from build123d import *

# Parameters (mm, degrees)
SKETCH1_R               = 16.6751
BOSS_EXTRUDE1_DEPTH     = 79.375
CUT_EXTRUDE1_DEPTH      = 83.804037009
CUT_EXTRUDE1_DEPTH_BACK = 83.804037009
SKETCH1_4_R             = 10.4648
SKETCH1_5_R             = 13.4366
SKETCH1_5_R_2           = 10.4648
CUT_EXTRUDE2_DEPTH      = 18.288
CUT_EXTRUDE3_START      = -18.288
SKETCH2_R               = 13.4366
SKETCH2_R_2             = 10.4648
CUT_EXTRUDE3_DEPTH      = 18.288
SKETCH3_R               = 13.5001
BOSS_EXTRUDE2_DEPTH     = 31.75
SKETCH3_7_R             = 7.8994
CUT_EXTRUDE5_DEPTH      = 33.3502
CUT_EXTRUDE6_START      = -17.526
SKETCH4_R               = 10.7696
SKETCH4_R_2             = 7.8994
CUT_EXTRUDE6_DEPTH      = 17.526
FILLET1_R               = 2.54


with BuildPart() as part:
    # Sketch1 → Boss-Extrude1 (new body)
    with BuildSketch(Plane(origin=(0, 0, 0), x_dir=(1, 0, 0), z_dir=(0, 1, 0))):
        with Locations(Location((0, 0, 0), (0, 0, 90))):
            Circle(SKETCH1_R)
    extrude(amount=BOSS_EXTRUDE1_DEPTH)

    # Sketch1<4> → Cut-Extrude1 (cut, two sides: drawn at the far end of the back side and taken through both)
    with BuildSketch(Plane(origin=(0, 0, 0), x_dir=(1, 0, 0), z_dir=(0, 1, 0)).offset(-CUT_EXTRUDE1_DEPTH_BACK)):
        with Locations(Location((0, 0, 0), (0, 0, 90))):
            Circle(SKETCH1_4_R)
    extrude(amount=CUT_EXTRUDE1_DEPTH + CUT_EXTRUDE1_DEPTH_BACK, mode=Mode.SUBTRACT)

    # Sketch1<5> → Cut-Extrude2 (cut)
    with BuildSketch(Plane(origin=(0, 0, 0), x_dir=(1, 0, 0), z_dir=(0, 1, 0))):
        with Locations(Location((0, 0, 0), (0, 0, 270))):
            Circle(SKETCH1_5_R)
        with Locations(Location((0, 0, 0), (0, 0, 90))):
            Circle(SKETCH1_5_R_2, mode=Mode.SUBTRACT)
    extrude(amount=CUT_EXTRUDE2_DEPTH, mode=Mode.SUBTRACT)

    # Sketch2 → Cut-Extrude3 (cut)
    with BuildSketch(Plane(origin=(0, 79.375, 0), x_dir=(1, 0, 0), z_dir=(0, 1, 0)).offset(CUT_EXTRUDE3_START)):
        with Locations(Location((0, 0, 0), (0, 0, 270))):
            Circle(SKETCH2_R)
        with Locations(Location((0, 0, 0), (0, 0, 90))):
            Circle(SKETCH2_R_2, mode=Mode.SUBTRACT)
    extrude(amount=CUT_EXTRUDE3_DEPTH, mode=Mode.SUBTRACT)

    # Sketch3 → Boss-Extrude2 (add)
    with BuildSketch(Plane(origin=(0, 0, 0), x_dir=(0, 0, -1), z_dir=(1, 0, 0))):
        with Locations(Location((0, 37.168433559, 0), (0, 0, 180))):
            Circle(SKETCH3_R)
    extrude(amount=BOSS_EXTRUDE2_DEPTH)

    # Sketch3<7> → Cut-Extrude5 (cut)
    with BuildSketch(Plane(origin=(0, 0, 0), x_dir=(0, 0, -1), z_dir=(1, 0, 0))):
        with Locations((0, 37.168433559)):
            Circle(SKETCH3_7_R)
    extrude(amount=CUT_EXTRUDE5_DEPTH, mode=Mode.SUBTRACT)

    # Sketch4 → Cut-Extrude6 (cut)
    with BuildSketch(Plane(origin=(31.75, 0, 0), x_dir=(0, 0, -1), z_dir=(1, 0, 0)).offset(CUT_EXTRUDE6_START)):
        with Locations((0, 37.168433559)):
            Circle(SKETCH4_R)
        with Locations((0, 37.168433559)):
            Circle(SKETCH4_R_2, mode=Mode.SUBTRACT)
    extrude(amount=CUT_EXTRUDE6_DEPTH, mode=Mode.SUBTRACT)

    # Fillet1
    fillet1_edges = [part.edges().sort_by_distance(p)[0] for p in [
        (9.788067225, 37.168433559, -13.5001),
    ]]
    fillet(fillet1_edges, radius=FILLET1_R)


solid = part.part
For this review, take the finished solid that the model builds, in its own axes (mm). A direction names the side the tool comes from. Give positions to 0.01 mm unless a question says otherwise; leave off trailing zeros. Order: outer loops, then holes, each group sorted by start corner. A loop starts at its lowest first (then second) coordinate and runs counter-clockwise, first axis right, second up. Notation, with made-up numbers: (4.25, 42.5) -> (42.25, 42.5) arc R33 cw to (42.25, 80.5) -> close; hole circle Ø5 at (-16, 32.5). An arc over 180 degrees is marked (long way). Write item = value, one per line.
1) We need section C-C, the plane x = -12. Give the boundary of the cut face in (y, z) (3 decimals), and give its area (3 significant figures).
Findings:
outline = (0, -11.578) -> (79.375, -11.578) -> (79.375, -6.045) -> (61.087, -6.045) -> (61.087, 6.045) -> (79.375, 6.045) -> (79.375, 11.578) -> (0, 11.578) -> (0, 6.045) -> (18.288, 6.045) -> (18.288, -6.045) -> (0, -6.045) -> close
area = 1,400 mm^2
2) Draft analysis for pull direction Z (two halves, no side actions). For faces 4 (the face through (-14, 79.375, -1)), 5 (the face through (-16.533, 39.132, 2.171)), 6 (the face through (-10.376, 39.388, 1.362)), state which applies: pulls with the +Z half, pulls with the -Z half, needs draft (parallel to the pull), parting line crosses it, or undercut.
Findings:
face_4 = needs draft
face_5 = parting line crosses it
face_6 = undercut
3) To check wall thickness, follow L1, parallel to Y at x = 10, z = 0; L2, parallel to X at y = 65.25, z = 0; L3, parallel to Y at x = -6.5, z = 10.5. State the ranges of each line that lie inside material, in increasing order. Write a range as from..to.
Findings:
L1 = 23.67..29.27, 45.07..50.67
L2 = -16.68..-13.44, 13.44..16.68
L3 = 18.29..61.09
4) Insertion check: pin 1 (2 mm diameter, centred on x = 18, y = 33.5, fed in from +Z); pin 2 (4 mm diameter, centred on x = 22, y = 24.5, fed in from -Z); pin 3 (1.5 mm diameter, centred on x = 1.5, z = -2.5, fed in from -Y). Each pin has a flat end and moves straight along its axis. Give the tip position at first contact, or say it passes through.
Findings:
pin_1 = 13.23
pin_2 = -8.27
pin_3 = 23.78
5) For faces 1 (the face through (0, 46, 0)), 2 (the face through (-8, 61.087, 7)), 3 (the face through (7.012, 30.16, -3.645)), list the 3-axis set-ups (+Z, -Z, +X, -X, +Y, -Y) from which the entire face can be reached by the end or side of a thin tool; tool diameter is ignored.
Findings:
face_1 = +Y, -Y
face_2 = +Y
face_3 = +X
6) We need section D-D, the plane x = 21. Give the boundary of the cut face in (y, z), and give its area (3 significant figures).
Findings:
outline = circle Ø27 at (37.17, 0); hole circle Ø21.54 at (37.17, 0)
area = 208 mm^2
7) We need section B-B, the plane y = 66. Give the boundary of the cut face in (x, z).
Findings:
outline = circle Ø33.35 at (0, 0); hole circle Ø26.87 at (0, 0)
8) We need section A-A, the plane z = 0. Count the separate pieces of the cut face and the enclosed holes in it, and give its area (3 significant figures).
Findings:
separate_pieces = 3
enclosed_holes = 0
area = 859 mm^2
